```python
from build123d import *

# Parameters (mm, degrees)
PAD008_DEPTH    = 40
POCKET019_DEPTH = 38
SKETCH042_R     = 2.35
POCKET020_DEPTH = 10
SKETCH044_R     = 1.4
POCKET023_DEPTH = 11
POCKET024_DEPTH = 52
FILLET001_R     = 1


with BuildPart() as part:
    # Sketch039 → Pad008 (new body, symmetric)
    with BuildSketch(Plane.YZ):
        Polygon((0, 70), (23, 70), (23, 0), (5, 0), (5, 52.3), (0, 57.3), align=None)
    extrude(amount=PAD008_DEPTH, both=True)

    # Sketch035 (on Face3 of Pad008) → Pocket019 (cut)
    with BuildSketch(Plane.YX):
        with BuildLine():
            ThreePointArc((-8.818597, 16.5), (-17.318597, 8), (-8.818597, -0.5))
            Line((-8.818597, -0.5), (9, -0.5))
            ThreePointArc((9, -0.5), (17.5, 8), (9, 16.5))
            Line((-8.818597, 16.5), (9, 16.5))
        make_face()
    extrude(amount=-POCKET019_DEPTH, mode=Mode.SUBTRACT)

    # Sketch042 (on Face1 of Pocket019) → Pocket020 (cut)
    with BuildSketch(Plane(origin=(0, 0, 70), x_dir=(0, -1, 0), z_dir=(0, 0, 1))):
        with Locations((-5, 30)):
            Circle(SKETCH042_R)
        with Locations((-5, -30)):
            Circle(SKETCH042_R)
    extrude(amount=-POCKET020_DEPTH, mode=Mode.SUBTRACT)

    # Sketch044 (on Face10 of Pocket020) → Pocket023 (cut)
    with BuildSketch(Plane(origin=(0, 5, 0), x_dir=(0, 0, -1), z_dir=(0, -1, 0))):
        with Locations((13, 30)):
            Circle(SKETCH044_R)
        with Locations((13, -30)):
            Circle(SKETCH044_R)
    extrude(amount=-POCKET023_DEPTH, mode=Mode.SUBTRACT)

    # Sketch048 (on Face12 of Pocket019) → Pocket024 (cut)
    with BuildSketch(Plane.YX.offset(-38)):
        with BuildLine():
            ThreePointArc((8, 13), (3, 8), (8, 3))
            Line((8, 3), (10, 3))
            ThreePointArc((10, 3), (15, 8), (10, 13))
            Line((8, 13), (10, 13))
        make_face()
    extrude(amount=-POCKET024_DEPTH, mode=Mode.SUBTRACT)

    # Fillet001
    fillet001_edges = [part.edges().sort_by_distance(p)[0] for p in [
        (12, 5, 45.15),
        (4, 5, 45.15),
    ]]
    fillet(fillet001_edges, radius=FILLET001_R)


solid = part.part
```
Check sheet for the modelled part. Datum: model origin and axes. Units: mm. A direction names the side the tool comes from. Round coordinates to 2 decimals unless told otherwise and drop trailing zeros. Loops run counter-clockwise (first coordinate to the right, second up) from the corner with the lowest first, then second, coordinate; pieces in that order, holes last. Notation, with made-up numbers: (56, 25.5) -> (96, 25.5) arc R29 ccw to (96, 54.5) -> close; hole circle Ø11 at (-28.75, 56.5). An arc over 180 degrees is marked (long way). Write item = value, one per line. Start each with the question number.
1) Set-up check for faces 5 (the flat face through (-30, 5, 60)), 6 (the flat face through (-0.5, 7, 19)), 7 (the flat face through (27, 5, 26)), 8 (the cylindrical face through (8, 3, 57)): record each of +Z, -Z, +X, -X, +Y, -Y from which the full face is reachable in a straight line by a thin tool's end or side.
2) Sectioned sample at C-C, the plane y = 16.5. Record the cut outline in (x, z), plus the area to 3 significant figures.
3) Release check for a two-part mould opening along X. For faces 1 (the flat face through (-40, 14, 35)), 2 (the flat face through (30, 5, 60)), 3 (the flat face through (16.5, 7, 19)), 4 (the flat face through (-19, 5, 26)) record: released by +X, released by -X, zero draft, split by the parting line, or undercut.
4) Sectioned sample at B-B, the plane x = -30. Record the cut outline in (y, z), plus the area to 3 significant figures.
5) Gauge pin test, flat ends, axial feed: pin 1 Ø8 at (x, z) = (27, 15) entering from -Y; pin 2 Ø2.5 at (x, y) = (29.5, 4.5) entering from +Z. Record the tip position at first contact, or that the pin passes through.
6) Sectioned sample at D-D, the plane x = 8.5. Record the cut outline in (y, z).
7) Thickness scan on probe 1 along X at (y, z) = (9.5, 51); probe 2 along X at (y, z) = (5.5, 67); probe 3 along X at (y, z) = (5.5, 19.5). Record the ranges inside material, lowest first.
8) Sectioned sample at A-A, the plane z = 7.5. Record the cut outline in (x, y).
Results are:
q1.face_5 = +Z
q1.face_6 = -Z, -Y
q1.face_7 = -Z, +X, -X, -Y
q1.face_8 = +Z, -Z
q2.outline = (-40, 0) -> (4, 0) -> (4, 38) -> (12, 38) -> (12, 0) -> (40, 0) -> (40, 70) -> (-40, 70) -> close
q2.area = 5,300 mm^2
q3.face_1 = released by -X
q3.face_2 = undercut
q3.face_3 = undercut
q3.face_4 = zero draft
q4.outline = (0, 57.3) -> (5, 52.3) -> (5, 0) -> (23, 0) -> (23, 70) -> (7.35, 70) -> (7.35, 60) -> (2.65, 60) -> (2.65, 70) -> (0, 70) -> close
q4.area = 1,290 mm^2
q5.pin_1 = 5
q5.pin_2 = 60
q6.outline = (0, 57.3) -> (3.03, 54.27) -> (3.03, 70) -> (0, 70) -> close; (14.97, 38) -> (17.49, 38) -> (17.49, 0) -> (23, 0) -> (23, 70) -> (14.97, 70) -> close
q7.probe_1 = -40 to 3, 13 to 40
q7.probe_2 = -40 to -32.3, -27.7 to 3.67, 12.33 to 27.7, 32.3 to 40
q7.probe_3 = -40 to -0.5, 16.5 to 40
q8.outline = (-40, 5) -> (-0.5, 5) -> (-0.5, 9) arc R8.5 cw to (16.5, 9) -> (16.5, 5) -> (40, 5) -> (40, 23) -> (-40, 23) -> close
